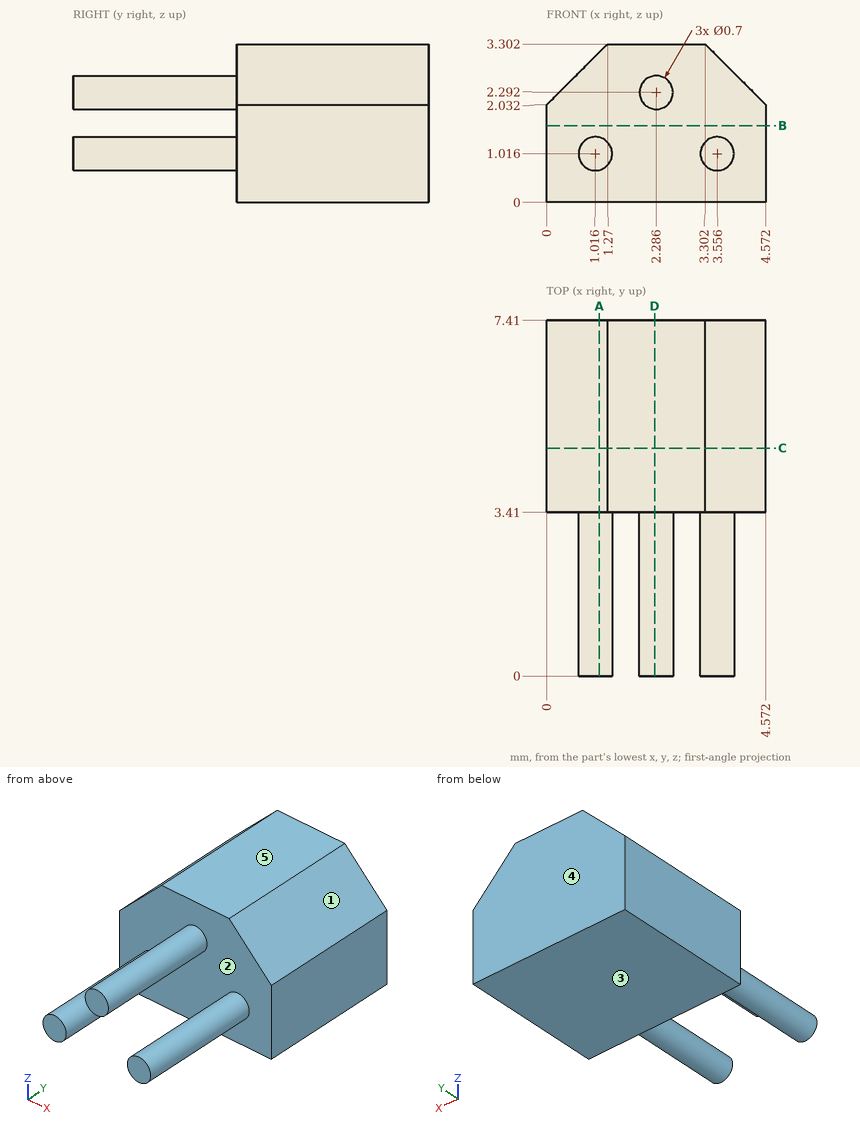
Can you work these out from the drawing? Everything is in mm from the part's minimum corner. A direction names the side the tool comes from. Round coordinates to 2 decimals unless told otherwise and drop trailing zeros. Write each loop counter-clockwise with the first axis right and the second up, starting at its lowest first coordinate (ties: lowest second). Pieces come first, ordered by that corner, then holes. Notation, with made-up numbers: M 63.5,57 L 111.5,57 A22 ccw 111.5,90 Z; hole C -34.75,-30.75 d6. An arc over 180 degrees is marked long. Use a Markdown table: item, result.
Item 1: Which directions (+Z, -Z, +X, -X, +Y, -Y) give clear straight access to the entire face, cutting with the end or side of a thin tool? Please do the marked faces 1 and 2.
Found:
| item | result |
|---|---|
| face 1 | +Z, +X, +Y, -Y |
| face 2 | -Y |
Item 2: I want a section at A-A (x = 1.1). List the corners of the cut face in (y, z) for me (1 decimal).
Found:
| item | result |
|---|---|
| outline | M 0,0.7 L 3.4,0.7 L 3.4,0 L 7.4,0 L 7.4,3.1 L 3.4,3.1 L 3.4,1.4 L 0,1.4 Z |
Item 3: I want a section at B-B (z = 1.6). List the corners of the cut face in (x, y) for me, and give its area (3 significant figures).
Found:
| item | result |
|---|---|
| outline | M 0,3.41 L 4.57,3.41 L 4.57,7.41 L 0,7.41 Z |
| area | 18.3 mm2 |
Item 4: If I drill on line 1 along Y through (x, z) = (3.25, 0.25); line 2 along X through (y, z) = (3, 2.3) (1 decimal); line 3 along Z through (x, y) = (3.6, 2.75), over which ranges is the centre line in solid material (lowest first)? Write a range as [from, to].
Found:
| item | result |
|---|---|
| line 1 | y = [3.41, 7.41] |
| line 2 | x = [1.9, 2.6] |
| line 3 | z = [0.67, 1.36] |
Item 5: I want a section at C-C (y = 4.75). List the corners of the cut face in (x, z) for me, and give its area (3 significant figures).
Found:
| item | result |
|---|---|
| outline | M 0,0 L 4.57,0 L 4.57,2.03 L 3.3,3.3 L 1.27,3.3 L 0,2.03 Z |
| area | 13.5 mm2 |
Item 6: We'd pull the mould along Z, two halves only. Please class the marked faces 3, 4 and 5: released by +Z, released by -Z, zero draft, split by the parting line, or undercut.
Found:
| item | result |
|---|---|
| face 3 | released by -Z |
| face 4 | zero draft |
| face 5 | released by +Z |
Item 7: I want a section at D-D (x = 2.25). List the corners of the cut face in (y, z) for me.
Found:
| item | result |
|---|---|
| outline | M 0,1.94 L 3.41,1.94 L 3.41,0 L 7.41,0 L 7.41,3.3 L 3.41,3.3 L 3.41,2.64 L 0,2.64 Z |
